Verification items for this drawing (mm, ordinates from the low corner). A direction names the side the tool comes from. Round coordinates to 2 decimals unless told otherwise and drop trailing zeros. Loops run counter-clockwise (first coordinate to the right, second up) from the corner with the lowest first, then second, coordinate; pieces in that order, holes last. Notation, with made-up numbers: (58, -32) - (74, -32) arc R21 ccw to (74, -24) - close; hole circle Ø4 at (18.5, 14.5). An arc over 180 degrees is marked (long way). Answer in a Markdown table with one row per item. Add a question column.
(1) Thickness scan on line 1 along Y through (x, z) = (4.5, 0.6); line 2 along Z through (x, y) = (8.75, 5.5); line 3 along Y through (x, z) = (12.5, 0.35). Record the ranges inside material, lowest first.
(2) Gauge pin test, flat ends, axial feed: pin 1 (1.5 mm diameter, centred on x = 3, z = 8, fed in from -Y); pin 2 (1.9 mm diameter, centred on y = 15, z = 32, fed in from +X); pin 3 (1.5 mm diameter, centred on y = 15.5, z = 23, fed in from -X). Record the tip position at first contact, or that the pin passes through.
(3) Mould release check, pull along Y, two halves, no side actions. Record for the marked faces 3, 4 and 5: +Y half, -Y half, draft (parallel to the pull), parting line (faces both ways), or undercut.
(4) Cross-section at D-D on z = 9. Enter the section's corners in (x, y).
(5) Cross-section at C-C on x = 14.5. Enter the section's corners in (y, z), then the cut area to 3 significant figures.
(6) Cross-section at A-A on y = 26. Enter the section's corners in (x, z), then the cut area to 3 significant figures.
(7) Access from +Z, -Z, +X, -X, +Y, -Y to the whole of each face (thin tool, end or side, straight path). Record for the marked faces 1 and 2.
(8) Cross-section at B-B on x = 8.5. Enter the section's corners in (y, z).
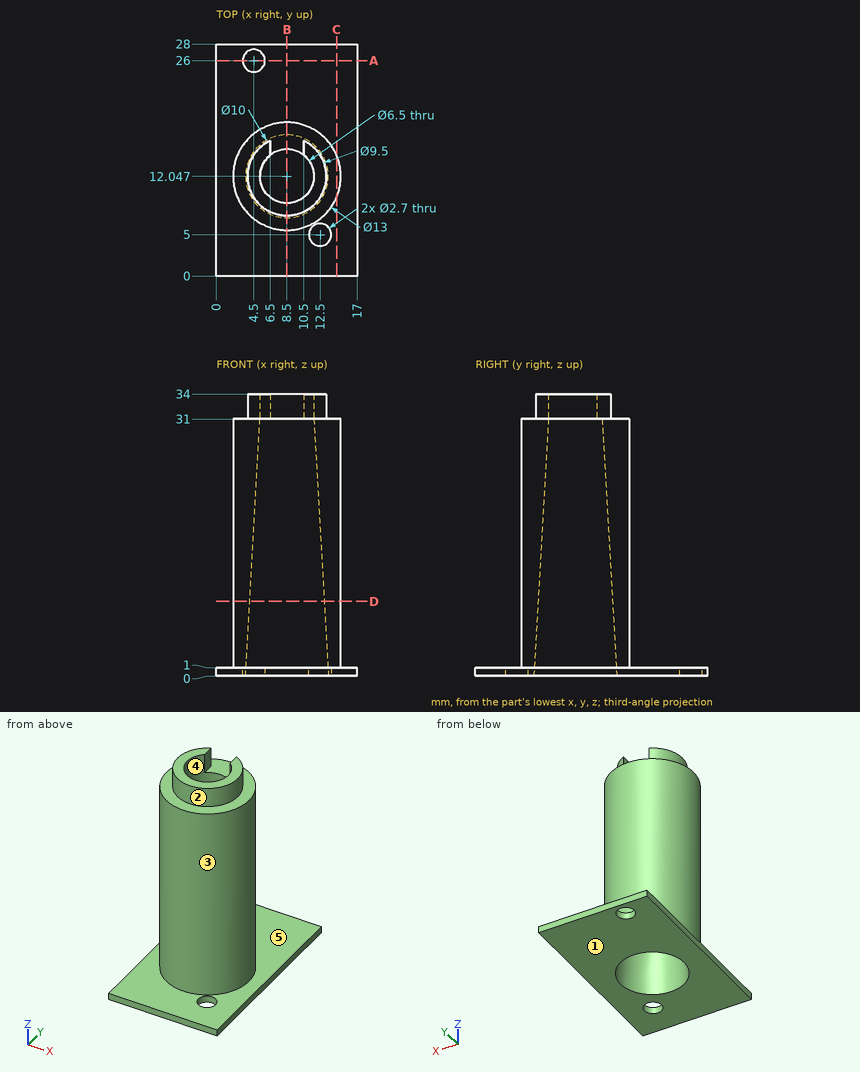
Answers:
| question | item | result |
|---|---|---|
| 1 | line 1 | y = 0 to 9.1, 14.99 to 24.65, 27.35 to 28 |
| 1 | line 2 | z = 0 to 1 |
| 1 | line 3 | y = 0 to 3.65, 6.35 to 9.08, 15.01 to 28 |
| 2 | pin 1 | stops at y = 7.61 |
| 2 | pin 2 | stops at x = 12.81 |
| 2 | pin 3 | stops at x = 2.59 |
| 3 | face 3 | parting line |
| 3 | face 4 | undercut |
| 3 | face 5 | draft |
| 4 | outline | circle Ø13 at (8.5, 12.05); hole circle Ø8.98 at (8.5, 12.05) |
| 5 | outline | (0, 0) - (28, 0) - (28, 1) - (14.55, 1) - (14.55, 31) - (9.55, 31) - (9.55, 1) - (0, 1) - close |
| 5 | area | 178 mm^2 |
| 6 | outline | (0, 0) - (3.15, 0) - (3.15, 1) - (0, 1) - close; (5.85, 0) - (17, 0) - (17, 1) - (5.85, 1) - close |
| 6 | area | 14.3 mm^2 |
| 7 | face 1 | -Z, +X, -X, +Y, -Y |
| 7 | face 2 | +Z |
| 8 | outline | (0, 0) - (7.05, 0) - (8.8, 31) - (8.8, 34) - (7.3, 34) - (7.3, 31) - (5.55, 31) - (5.55, 1) - (0, 1) - close; (15.3, 31) - (17.05, 0) - (28, 0) - (28, 1) - (18.55, 1) - (18.55, 31) - close |
